Geometry check sheet. Reference: the model listing, model coordinates, mm. Face numbers are marked on the shaded views. A direction names the side the tool comes from. Round coordinates to 2 decimals unless told otherwise and drop trailing zeros. Write each loop counter-clockwise with the first axis right and the second up, starting at its lowest first coordinate (ties: lowest second). Pieces come first, ordered by that corner, then holes.
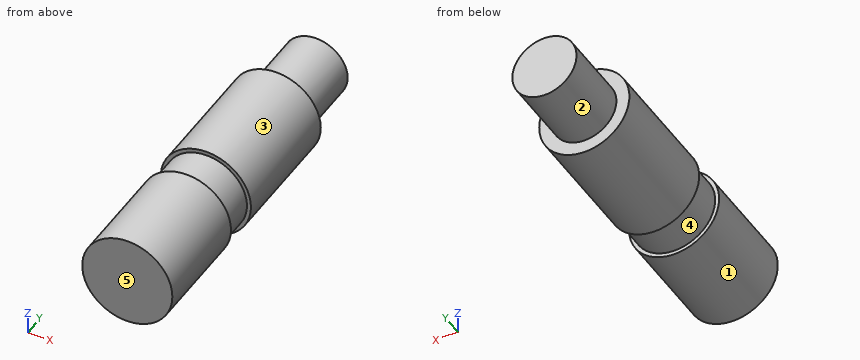
from build123d import *

# Parameters (mm, degrees)
SKETCH1_R           = 15.875
BOSS_EXTRUDE1_DEPTH = 119.888
SKETCH2_R           = 15.875
SKETCH2_R_2         = 11.303
CUT_EXTRUDE1_DEPTH  = 25.4
CUT_EXTRUDE2_START  = -69.85
SKETCH3_R           = 15.875
SKETCH3_R_2         = 14.478
CUT_EXTRUDE2_DEPTH  = 12.7


with BuildPart() as part:
    # Sketch1 → Boss-Extrude1 (new body)
    with BuildSketch(Plane(origin=(0, 0, 0), x_dir=(1, 0, 0), z_dir=(0, 1, 0))):
        Circle(SKETCH1_R)
    extrude(amount=BOSS_EXTRUDE1_DEPTH)

    # Sketch2 → Cut-Extrude1 (cut)
    with BuildSketch(Plane(origin=(0, 119.888, 0), x_dir=(1, 0, 0), z_dir=(0, 1, 0))):
        Circle(SKETCH2_R)
        Circle(SKETCH2_R_2, mode=Mode.SUBTRACT)
    extrude(amount=-CUT_EXTRUDE1_DEPTH, mode=Mode.SUBTRACT)

    # Sketch3 → Cut-Extrude2 (cut)
    with BuildSketch(Plane(origin=(0, 119.888, 0), x_dir=(1, 0, 0), z_dir=(0, 1, 0)).offset(CUT_EXTRUDE2_START)):
        Circle(SKETCH3_R)
        Circle(SKETCH3_R_2, mode=Mode.SUBTRACT)
    extrude(amount=-CUT_EXTRUDE2_DEPTH, mode=Mode.SUBTRACT)


solid = part.part
1. Section check D-D (x = -13). Record the cut outline in (y, z), plus the area to 3 significant figures.
2. Release check for a two-part mould opening along Y. For the marked faces 3, 4 and 5 record: +Y half, -Y half, draft (parallel to the pull), parting line (faces both ways), or undercut.
3. Depth check by flat-ended pin: pin 1 Ø1 at (x, y) = (-9.5, 82.5) entering from +Z; pin 2 Ø3 at (x, y) = (-9.5, 101) entering from +Z; pin 3 Ø8 at (y, z) = (21.5, -4.5) entering from -X. Enter the tip coordinate at first touch or a pass-through.
4. Section check C-C (y = 66). Record the cut outline in (x, z) (3 decimals), plus the area to 3 significant figures.
5. Scan lines: line 1 along Y through (x, z) = (13, -7); line 2 along Y through (x, z) = (-1, 13.5); line 3 along Z through (x, y) = (0.5, 23). Record each from-to range of solid material in increasing order.
6. Access from +Z, -Z, +X, -X, +Y, -Y to the whole of each face (thin tool, end or side, straight path). Record for the marked faces 1 and 2.
7. Section check A-A (z = 0). Record the cut outline in (x, y) (3 decimals).
8. Section check B-B (x = 0). Record the cut outline in (y, z) (3 decimals), plus the area to 3 significant figures.
Results below:
1. outline: (0, -9.11) - (37.34, -9.11) - (37.34, -6.37) - (50.04, -6.37) - (50.04, -9.11) - (94.49, -9.11) - (94.49, 9.11) - (50.04, 9.11) - (50.04, 6.37) - (37.34, 6.37) - (37.34, 9.11) - (0, 9.11) - close
1. area: 1,650 mm2
2. face 3: draft
2. face 4: undercut
2. face 5: -Y half
3. pin 1: stops at z = 13.08
3. pin 2: stops at z = 7.98
3. pin 3: stops at x = -15.87
4. outline: circle Ø31.75 at (0, 0)
4. area: 792 mm2
5. line 1: y = 0 to 37.34, 50.04 to 94.49
5. line 2: y = 0 to 94.49
5. line 3: z = -15.87 to 15.87
6. face 1: +Y, -Y
6. face 2: +Y
7. outline: (-15.875, 0) - (15.875, 0) - (15.875, 37.338) - (14.478, 37.338) - (14.478, 50.038) - (15.875, 50.038) - (15.875, 94.488) - (11.303, 94.488) - (11.303, 119.888) - (-11.303, 119.888) - (-11.303, 94.488) - (-15.875, 94.488) - (-15.875, 50.038) - (-14.478, 50.038) - (-14.478, 37.338) - (-15.875, 37.338) - close
8. outline: (0, -15.875) - (37.338, -15.875) - (37.338, -14.478) - (50.038, -14.478) - (50.038, -15.875) - (94.488, -15.875) - (94.488, -11.303) - (119.888, -11.303) - (119.888, 11.303) - (94.488, 11.303) - (94.488, 15.875) - (50.038, 15.875) - (50.038, 14.478) - (37.338, 14.478) - (37.338, 15.875) - (0, 15.875) - close
8. area: 3,540 mm2
